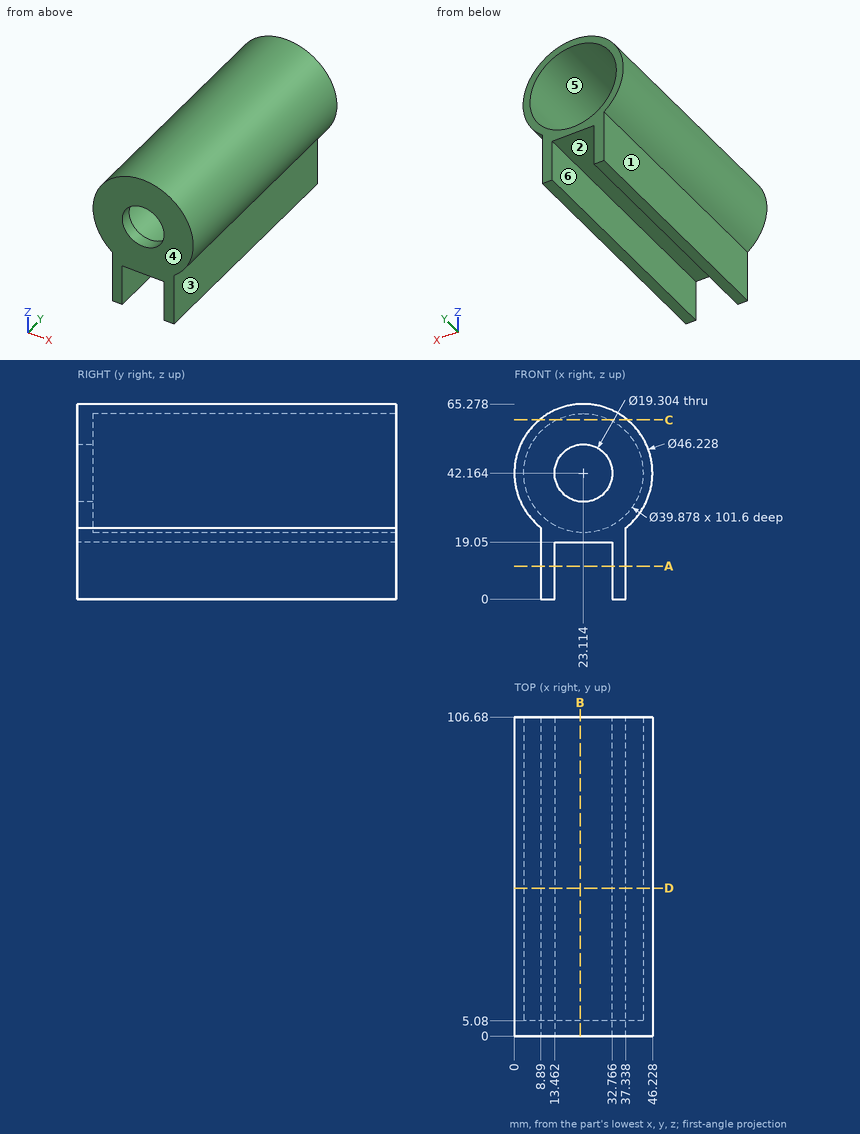
Part print with two shaded views. Sizes in mm from the minimum x, y, z corner. A direction names the side the tool comes from. Coordinates: 2 decimals unless noted, no trailing zeros. Write each loop counter-clockwise with the first axis right and the second up, starting at its lowest first coordinate (ties: lowest second). Pieces come first, ordered by that corner, then holes. Notation, with made-up numbers: M -31.75,-20 L 24.25,-20 A22 cw 24.25,18 Z; hole C 15,42.5 d3. An arc over 180 degrees is marked long. Return JSON: item names as keys, results as strings.
Item 1: Which spindle directions (+Z, -Z, +X, -X, +Y, -Y) get a long thin tool onto all of the face, cutting with end or side? Do the marked faces 4, 5 and 6. Say none if no direction does.
Findings below:
{"face 4": "+Z, -Z, +X, -X, -Y", "face 5": "+Y", "face 6": "-Z, +Y, -Y"}
Item 2: Drop flat-ended pins along their axis: pin 1 Ø12 at (y, z) = (38.5, 49) entering from -X; pin 2 Ø5 at (y, z) = (77, 16.5) entering from -X; pin 3 Ø9.5 at (y, z) = (66.5, 8) entering from +X. Give the stop position or say it passes through.
Findings below:
{"pin 1": "stops at x = 0.02", "pin 2": "stops at x = 8.89", "pin 3": "stops at x = 37.34"}
Item 3: Slice it at C-C, the plane z = 60. Write the cut outline in (x, y).
Findings below:
{"outline": "M 8.41,0 L 37.82,0 L 37.82,106.68 L 32.03,106.68 L 32.03,5.08 L 14.2,5.08 L 14.2,106.68 L 8.41,106.68 Z"}
Item 4: Two-plate mould, pull along X, no slides. Class the marked faces 1, 2 and 3: +X half, -X half, draft (parallel to the pull), parting line (faces both ways), or undercut.
Findings below:
{"face 1": "-X half", "face 2": "undercut", "face 3": "+X half"}
Item 5: Probe line 1 (X direction, y = 65.5, z = 12); line 2 (Z direction, x = 24, y = 75); line 3 (X direction, y = 100, z = 21). List the from-to ranges inside material, lowest first. Write a range as from..to.
Findings below:
{"line 1": "x = 8.89..13.46, 32.77..37.34", "line 2": "z = 19.05..22.24, 62.08..65.26", "line 3": "x = 8.89..37.34"}
Item 6: Slice it at B-B, the plane x = 22. Write the cut outline in (y, z), and give its area (3 significant figures).
Findings below:
{"outline": "M 0,19.05 L 106.68,19.05 L 106.68,22.26 L 5.08,22.26 L 5.08,32.58 L 0,32.58 Z; M 0,51.75 L 5.08,51.75 L 5.08,62.07 L 106.68,62.07 L 106.68,65.25 L 0,65.25 Z", "area": "786 mm2"}
Item 7: Slice it at A-A, the plane z = 11. Write the cut outline in (x, y), and give its area (3 significant figures).
Findings below:
{"outline": "M 8.89,0 L 13.46,0 L 13.46,106.68 L 8.89,106.68 Z; M 32.77,0 L 37.34,0 L 37.34,106.68 L 32.77,106.68 Z", "area": "975 mm2"}
Item 8: Slice it at D-D, the plane y = 49.5. Write the cut outline in (x, z).
Findings below:
{"outline": "M 8.89,0 L 13.46,0 L 13.46,19.05 L 32.77,19.05 L 32.77,0 L 37.34,0 L 37.34,23.94 A23.11 ccw long 8.89,23.94 Z; hole C 23.11,42.16 d39.88"}
